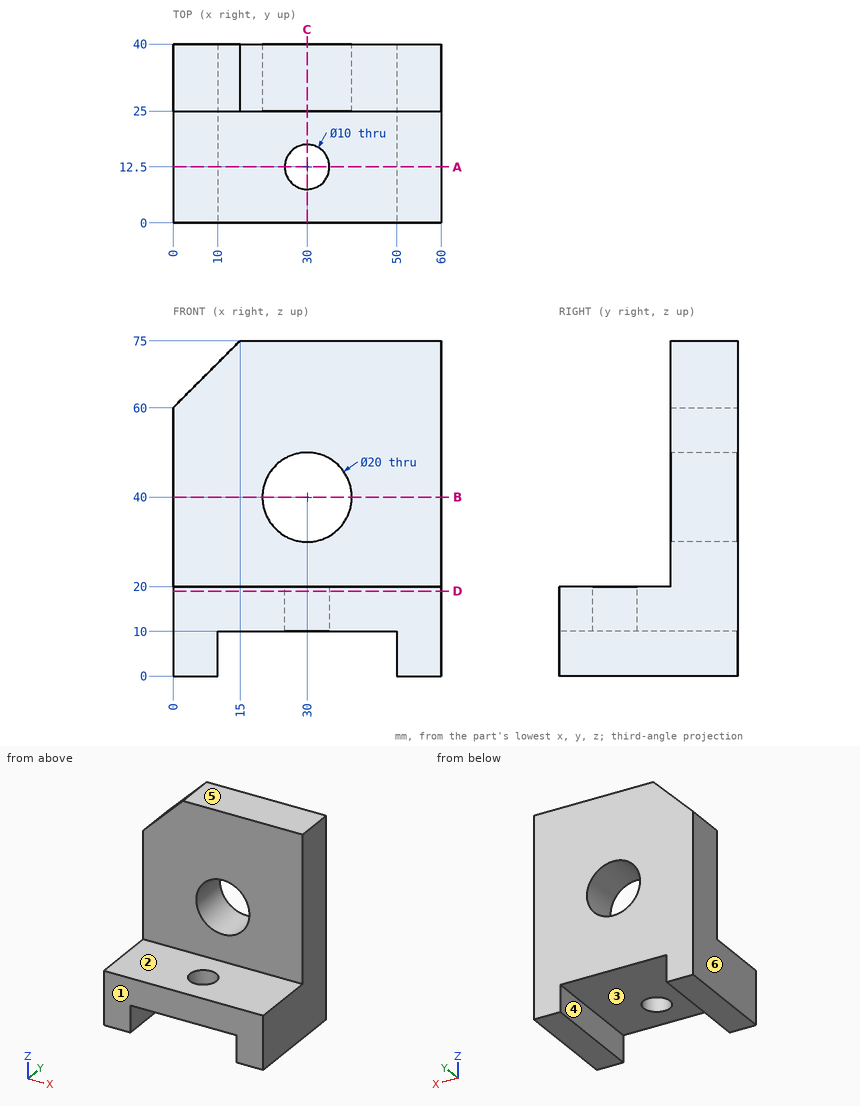
Could you check a few things on this drawing? It's one solid part, dimensions in mm from its lowest x, y, z. A direction names the side the tool comes from. Coordinates: 2 decimals unless noted, no trailing zeros. Write each loop counter-clockwise with the first axis right and the second up, starting at its lowest first coordinate (ties: lowest second). Pieces come first, ordered by that corner, then holes. Notation, with made-up numbers: (-22, -39) - (1, -39) arc R17 cw to (1, -28) - close; hole circle Ø5 at (4, 47.5). An arc over 180 degrees is marked (long way). Return JSON: item names as keys, results as strings. Group by question number.
Item 1: Which directions (+Z, -Z, +X, -X, +Y, -Y) give clear straight access to the entire face, cutting with the end or side of a thin tool? Please do the marked faces 1, 2 and 3.
Item 2: If we section it at B-B (z = 40): Write out the boundary of the cut face in (x, y), then the cut area to 3 significant figures.
Item 3: We'd pull the mould along X, two halves only. Please class the marked faces 4, 5 and 6: pulls with the +X half, pulls with the -X half, needs draft (parallel to the pull), parting line crosses it, or undercut.
Item 4: Please list where these lines run through material, in increasing order: probe 1 along Y at (x, z) = (30, 13.25); probe 2 along Z at (x, y) = (19.5, 37); probe 3 along Y at (x, z) = (43, 40.5).
Item 5: If we section it at C-C (x = 30): Write out the boundary of the cut face in (y, z).
Item 6: I'm going to push flat-ended pins straight in: pin 1 Ø6 at (x, y) = (30, 12.5) entering from +Z; pin 2 Ø8 at (x, z) = (17.5, 52) entering from -Y; pin 3 Ø1.5 at (x, y) = (7.5, 34) entering from +Z; pin 4 Ø20 at (x, y) = (29, 29) entering from -Z. Where does each tip first touch, or does it pass through?
Item 7: If we section it at A-A (y = 12.5): Write out the boundary of the cut face in (x, z), then the cut area to 3 significant figures.
Item 8: If we section it at D-D (z = 19): Write out the boundary of the cut face in (x, y), then the cut area to 3 significant figures.
Return value:
{
 "1": {"face 1": "+Z, -Z, +X, -X, -Y", "face 2": "+Z, +X, -X, -Y", "face 3": "-Z, +Y, -Y"},
 "2": {"outline": "(0, 25) - (20, 25) - (20, 40) - (0, 40) - close; (40, 25) - (60, 25) - (60, 40) - (40, 40) - close", "area": "600 mm^2"},
 "3": {"face 4": "undercut", "face 5": "needs draft", "face 6": "pulls with the -X half"},
 "4": {"probe 1": "y = 0 to 7.5, 17.5 to 40", "probe 2": "z = 10 to 75", "probe 3": "y = 25 to 40"},
 "5": {"outline": "(0, 10) - (7.5, 10) - (7.5, 20) - (0, 20) - close; (17.5, 10) - (40, 10) - (40, 30) - (25, 30) - (25, 20) - (17.5, 20) - close; (25, 50) - (40, 50) - (40, 75) - (25, 75) - close"},
 "6": {"pin 1": "passes through", "pin 2": "stops at y = 25", "pin 3": "stops at z = 68.25", "pin 4": "stops at z = 10"},
 "7": {"outline": "(0, 0) - (10, 0) - (10, 10) - (25, 10) - (25, 20) - (0, 20) - close; (35, 10) - (50, 10) - (50, 0) - (60, 0) - (60, 20) - (35, 20) - close", "area": "700 mm^2"},
 "8": {"outline": "(0, 0) - (60, 0) - (60, 40) - (0, 40) - close; hole circle Ø10 at (30, 12.5)", "area": "2,320 mm^2"}
}
